```python
from build123d import *

# Parameters (mm, degrees)
SKETCH1_R           = 10
SKETCH1_R_2         = 5
BOSS_EXTRUDE1_DEPTH = 10
CHAMFER1_SIZE       = 1
SKETCH3_W           = 1.65
SKETCH3_H           = 10
CIRPATTERN1_COUNT   = 3


with BuildPart() as part:
    # Sketch1 → Boss-Extrude1 (new body)
    with BuildSketch(Plane(origin=(0, 0, 0), x_dir=(1, 0, 0), z_dir=(0, 1, 0))):
        with Locations(Location((0, 0, 0), (0, 0, 270))):
            Circle(SKETCH1_R)
        with Locations(Location((0, 0, 0), (0, 0, 270))):
            Circle(SKETCH1_R_2, mode=Mode.SUBTRACT)
    extrude(amount=-BOSS_EXTRUDE1_DEPTH)

    # Chamfer1
    chamfer1_edges = [part.edges().sort_by_distance(p)[0] for p in [
        (0, 0, -10),
        (0, -10, -10),
        (0, -10, -5),
        (0, 0, -5),
    ]]
    chamfer(chamfer1_edges, length=CHAMFER1_SIZE)

    # Sketch3 → M4 Tapped Hole1 (revolve, cut)
    with BuildSketch(Plane(origin=(0, -5, 0), x_dir=(0, 1, 0), z_dir=(1, 0, 0))):
        with Locations((0.825, 5)):
            Rectangle(SKETCH3_W, SKETCH3_H)
    m4_tapped_hole1 = revolve(axis=Axis((0, -5, -6.35), (0, 0, 1)), mode=Mode.SUBTRACT)

    # CirPattern1: M4 Tapped Hole1 ×3 about axis
    cirpattern1_axis = Axis((0, -1, 0), (0, 1, 0))
    for i in range(1, CIRPATTERN1_COUNT):
        add(m4_tapped_hole1.rotate(cirpattern1_axis, i * 360 / CIRPATTERN1_COUNT), mode=Mode.SUBTRACT)


solid = part.part
```
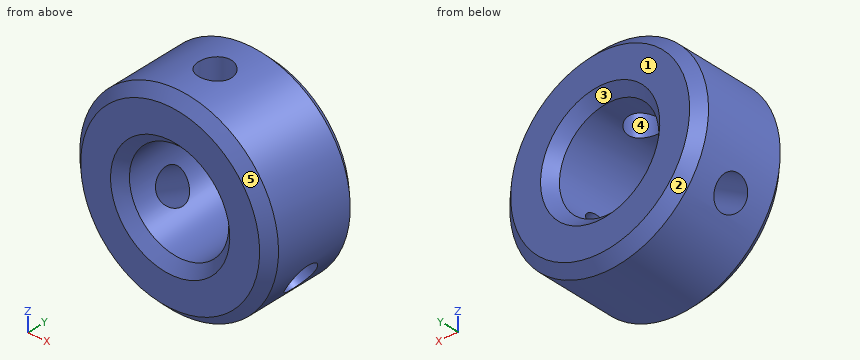
Design review of the part built by this model. Coordinates are the model's own, in mm. Face numbers are marked on the shaded views. A direction names the side the tool comes from. Give positions to 0.01 mm unless a question says otherwise; leave off trailing zeros. Loops run counter-clockwise (first coordinate to the right, second up) from the corner with the lowest first, then second, coordinate; pieces in that order, holes last. Notation, with made-up numbers: M 28.25,-20.5 L 59.25,-20.5 A30 ccw 59.25,18.5 Z; hole C 51.25,43.5 d10. An arc over 180 degrees is marked long. Return JSON: item names as keys, results as strings. Group by question number.
Item 1: We need section D-D (y = -5). Give the boundary of the cut face in (x, z).
Item 2: Tool access review of the marked faces 4 and 5: name each direction out of +Z, -Z, +X, -X, +Y, -Y from which nothing blocks a thin tool from reaching the whole face with its end or side.
Item 3: We need section A-A (x = 0). Give the boundary of the cut face in (y, z).
Item 4: Insertion check: pin 1 Ø5 at (x, y) = (-5.5, -2.5) entering from -Z; pin 2 Ø2 at (x, y) = (0, -5) entering from +Z; pin 3 Ø2 at (y, z) = (-4, -4.5) entering from -X. Each pin has a flat end and moves straight along its axis. Give the tip position at first contact, or say it passes through.
Item 5: We need section B-B (z = 0). Give the boundary of the cut face in (x, y).
Item 6: We need section C-C (y = -2). Give the boundary of the cut face in (x, z), and give its area (3 significant figures).
Item 7: For probe 1 along Y at (x, z) = (0, 8.5); probe 2 along X at (y, z) = (-3.25, 0); probe 3 along Z at (x, y) = (-5.75, -4.75), list the stretches that pass through material, from the lowest coordinate up.
Item 8: Mouldability with a two-part tool opening along Z and no side actions: class the marked faces 1, 2 and 3 as released by +Z, released by -Z, zero draft, split by the parting line, or undercut.
Output:
{
 "1": {"outline": "M -9.37,-3.5 L -4.91,-0.93 A5 cw -1.65,4.72 L -1.65,9.86 A10 ccw Z; M -7.72,-6.36 A10 ccw 7.72,-6.36 L 3.26,-3.79 A5 cw -3.26,-3.79 Z; M 1.65,4.72 A5 cw 4.91,-0.93 L 9.37,-3.5 A10 ccw 1.65,9.86 Z"},
 "2": {"face 4": "+Z", "face 5": "-Y"},
 "3": {"outline": "M -10,-9 L -9,-10 L -1,-10 L 0,-9 L 0,-6 L -1,-5 L -9,-5 L -10,-6 Z; M -10,6 L -9,5 L -6.65,5 L -6.65,10 L -9,10 L -10,9 Z; M -3.35,5 L -1,5 L 0,6 L 0,9 L -1,10 L -3.35,10 Z"},
 "4": {"pin 1": "stops at z = -9.54", "pin 2": "stops at z = -4.9", "pin 3": "stops at x = -9.37"},
 "5": {"outline": "M -10,-9 L -9,-10 L -6,-10 L -5,-9 L -5,-1 L -6,0 L -9,0 L -10,-1 Z; M 5,-9 L 6,-10 L 9,-10 L 10,-9 L 10,-1 L 9,0 L 6,0 L 5,-1 Z"},
 "6": {"outline": "C 0,0 d20; hole C 0,0 d10", "area": "236 mm^2"},
 "7": {"probe 1": "y = -10 to -6.65, -3.35 to 0", "probe 2": "x = -10 to -5, 5 to 10", "probe 3": "z = -8.18 to -5.2, -1.44 to 8.18"},
 "8": {"face 1": "zero draft", "face 2": "split by the parting line", "face 3": "undercut"}
}
